For this review, take the finished solid that the model builds, in its own axes (mm). A direction names the side the tool comes from. Coordinates: 2 decimals unless noted, no trailing zeros. Order: outer loops, then holes, each group sorted by start corner. A loop starts at its lowest first (then second) coordinate and runs counter-clockwise, first axis right, second up. Notation, with made-up numbers: (-17, -27.75) -> (24, -27.75) arc R13 cw to (24, -17.75) -> close; hole circle Ø5 at (-12.5, 2). An arc over 180 degrees is marked (long way). Return JSON: item names as keys, results as strings. Group by question number.
Item 1: Insertion check: pin 1 (5 mm diameter, centred on y = 16, z = -12.5, fed in from -X); pin 2 (11.5 mm diameter, centred on x = 0, z = 0, fed in from +Y); pin 3 (1 mm diameter, centred on y = 32, z = 25, fed in from -X); pin 4 (12 mm diameter, centred on x = -14, y = 38, fed in from -Z). Each pin has a flat end and moves straight along its axis. Give the tip position at first contact, or say it passes through.
Item 2: Take a section at C-C (x = 48). Write out the cut boundary in (y, z).
Item 3: For line 1 along X through (y, z) = (36.5, 0) (3 decimals); line 2 along Z through (x, y) = (0, 35.75) (3 decimals); line 3 along X through (y, z) = (14.5, -15), list the stretches that pass through material, from the lowest coordinate up.
Item 4: Draft analysis for pull direction X (two halves, no side actions). For faces 5 (the flat face through (69.85, 22, 0)), 6 (the flat face through (0, 41, -32)), 7 (the flat face through (44.45, 22, 14)), state which applies: +X half, -X half, draft (parallel to the pull), parting line (faces both ways), or undercut.
Item 5: Machinability: for faces 1 (the flat face through (49.212, 22, -13)), 2 (the flat face through (35, 22, 15.875)), 3 (the flat face through (0, 31.75, 0)), 4 (the flat face through (35, 22, -15.875)), which of the approach directions +Z, -Z, +X, -X, +Y, -Y give a long, thin tool a straight path to every point of the face, cutting with its end or side? Answer none if there is none.
Item 6: Take a section at B-B (z = 0). Write out the cut boundary in (x, y) (3 decimals).
Autodesk Inventor part; units mm, degrees
ref_plane "YZ Plane" through (0, 0, 0) normal (1, 0, 0) x (0, 1, 0)
ref_plane "XZ Plane" through (0, 0, 0) normal (0, 1, 0) x (-1, 0, 0)
ref_plane "XY Plane" through (0, 0, 0) normal (0, 0, 1) x (1, 0, 0)
sketch "Boceto1" plane through (0, 0, 0) normal (0, 1, 0) x (-1, 0, 0)
  line L0 (25.4, 44.45) -> (-25.4, 44.45)
  line L1 (-25.4, 44.45) -> (-25.4, -44.45)
  line L2 (-25.4, -44.45) -> (25.4, -44.45)
  line L3 (25.4, -44.45) -> (25.4, 44.45)
  line L4 (25.4, 44.45) -> (-25.4, -44.45) construction
  line L5 (-25.4, 44.45) -> (25.4, -44.45) construction
  line L6 (-25.4, -15.875) -> (-69.85, -15.875)
  line L7 (-69.85, -15.875) -> (-69.85, 15.875)
  line L8 (-69.85, 15.875) -> (-25.4, 15.875)
  line L9 (-25.4, 15.875) -> (-25.4, -15.875)
  line L10 (-25.4, 44.45) -> (0, 44.45)
  line L11 (0, 44.45) -> (0, -44.45)
  line L12 (0, -44.45) -> (-25.4, -44.45)
  line L13 (-25.4, -44.45) -> (-25.4, 44.45)
  line L14 (-25.4, 15.875) -> (-43.4008, 15.875)
  line L15 (-25.4, 15.875) -> (-44.45, 15.875)
  line L16 (-44.45, 15.875) -> (-49.2125, 15.875)
  line L17 (-49.2125, 15.875) -> (-44.45, 15.875)
  line L18 (-44.45, 15.875) -> (-44.45, 11.1125)
  line L19 (-44.45, 11.1125) -> (-49.2125, 11.1125)
  line L20 (-49.2125, 11.1125) -> (-49.2125, 15.875)
  line L21 (-49.2125, -15.875) -> (-44.45, -15.875)
  line L22 (-44.45, -15.875) -> (-44.45, -11.1125)
  line L23 (-44.45, -11.1125) -> (-49.2125, -11.1125)
  line L24 (-49.2125, -11.1125) -> (-49.2125, -15.875)
  point P0 (0, 0)
  dimension "d0" = 28.575
  dimension "d1" = 28.575
  dimension "d2" = 31.75
  dimension "d3" = 50.8
  dimension "d4" = 44.45
  dimension "d5" = 19.05
  dimension "d6" = 4.7625
  dimension "d7" = 4.7625
  dimension "d8" = 4.7625
  dimension "d9" = 4.7625
  dimension "d10" = 19.05
extrude "Extrusión1" add sketch "Boceto1" along normal blind 44.45 contours L11 L2 L1 L0 | L1 L6 L22 L23 L24 L7 L8 L20 L19 L18
sketch "Boceto2" plane through (0, 0, 44.45) normal (0, 0, 1) x (1, 0, 0)
  line L0 (0, 0) -> (25.4, 0)
  line L1 (25.4, 0) -> (9.525, 0)
  circle A0 centre (9.525, 0) radius 38.1
  line L2 (25.4, 0) -> (-25.4, 0)
  line L3 (-25.4, 0) -> (-25.4, 15.2268)
  line L4 (0, 0) -> (0, 36.8902)
  dimension "d13" = 15.875
  dimension "d14" = 76.2
  dimension "d15" = 50.8
extrude "Extrusión2" add sketch "Boceto2" against normal blind 88.9 contours L4 L2 L3 A0 picked at (-16.9333, 5.0756)
sketch "Boceto3" plane through (0, 44.45, 0) normal (0, 1, 0) x (1, 0, 0)
  circle A0 centre (0, 0) radius 19.05
  circle A1 centre (0, 0) radius 9.525
  dimension "d18" = 38.1
  dimension "d19" = 19.05
extrude "Extrusión3" add sketch "Boceto3" against normal blind 25.4
sketch "Boceto4" plane through (0, 44.45, 0) normal (0, 1, 0) x (1, 0, 0)
  circle A0 centre (0, 0) radius 9.525
  dimension "d22" = 19.05
extrude "Extrusión4" cut sketch "Boceto4" against normal blind 12.7
properties part number "Pieza6-Tarea1"
Findings below:
{
 "1": {"pin 1": "stops at x = -25.4", "pin 2": "stops at y = 31.75", "pin 3": "stops at x = -11.91", "pin 4": "stops at z = -17.29"},
 "2": {"outline": "(0, -11.11) -> (44.45, -11.11) -> (44.45, 11.11) -> (0, 11.11) -> close"},
 "3": {"line 1": "x = -19.05 to -9.525, 9.525 to 69.85", "line 2": "z = -44.45 to -9.525, 9.525 to 44.45", "line 3": "x = -25.4 to 44.45, 49.21 to 69.85"},
 "4": {"face 5": "+X half", "face 6": "-X half", "face 7": "undercut"},
 "5": {"face 1": "-Z, +Y, -Y", "face 2": "+Z, +X, +Y, -Y", "face 3": "+Y", "face 4": "-Z, +X, +Y, -Y"},
 "6": {"outline": "(-25.4, 0) -> (69.85, 0) -> (69.85, 44.45) -> (9.525, 44.45) -> (9.525, 31.75) -> (-9.525, 31.75) -> (-9.525, 44.45) -> (-19.05, 44.45) -> (-19.05, 25.201) arc R38.1 ccw to (-25.4, 15.227) -> close"}
}
